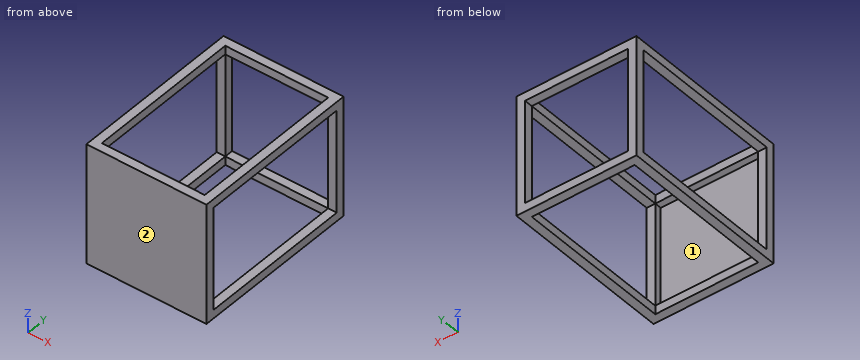
Autodesk Inventor part; units mm, degrees
ref_plane "YZ Plane" through (0, 0, 0) normal (1, 0, 0) x (0, 1, 0)
ref_plane "XZ Plane" through (0, 0, 0) normal (0, 1, 0) x (-1, 0, 0)
ref_plane "XY Plane" through (0, 0, 0) normal (0, 0, 1) x (1, 0, 0)
sketch "Sketch1" plane through (0, 0, 0) normal (0, 0, 1) x (1, 0, 0)
  point P0 (0, 0)
sketch "Sketch2" plane through (0, 0, 0) normal (0, 1, 0) x (-1, 0, 0)
  line L0 (-300, 300) -> (300, 300)
  line L1 (300, 300) -> (300, -300)
  line L2 (300, -300) -> (-300, -300)
  line L3 (-300, -300) -> (-300, 300)
  line L4 (-300, 300) -> (300, -300) construction
  line L5 (300, 300) -> (-300, -300) construction
  line L6 (350, 350) -> (-350, 350)
  line L7 (-350, 350) -> (-350, -350)
  line L8 (-350, -350) -> (350, -350)
  line L9 (350, -350) -> (350, 350)
  line L10 (350, 350) -> (-350, -350) construction
  line L11 (-350, 350) -> (350, -350) construction
  line L12 (-300, 300) -> (-350, 300)
  line L13 (-350, 300) -> (-350, 350)
  line L14 (-350, 350) -> (-300, 350)
  line L15 (-300, 350) -> (-300, 300)
  line L16 (300, 300) -> (350, 300)
  line L17 (350, 300) -> (350, 350)
  line L18 (350, 350) -> (300, 350)
  line L19 (300, 350) -> (300, 300)
  line L20 (350, -350) -> (300, -350)
  line L21 (300, -350) -> (300, -300)
  line L22 (300, -300) -> (350, -300)
  line L23 (350, -300) -> (350, -350)
  line L24 (-350, -350) -> (-300, -350)
  line L25 (-300, -350) -> (-300, -300)
  line L26 (-300, -300) -> (-350, -300)
  line L27 (-350, -300) -> (-350, -350)
  point P0 (0, 0)
  dimension "d0" = 600
  dimension "d1" = 600
  dimension "d2" = 700
  dimension "d3" = 700
extrude "Extrusion1" add sketch "Sketch2" along normal blind 10 contours L0 L1 L2 L3
extrude "Extrusion2" add sketch "Sketch2" along normal blind 50 contours L15 L6 L19 L0 | L3 L26 L7 L12 | L12 L7 L6 L15 | L16 L9 L22 L1 | L19 L6 L9 L16 | L2 L21 L8 L25 | L25 L8 L7 L26 | L22 L9 L8 L21
extrude "Extrusion3" add sketch "Sketch2" along normal blind 1000 contours L12 L7 L6 L15 | L19 L6 L9 L16 | L25 L8 L7 L26 | L22 L9 L8 L21
sketch3d "3D Sketch1"
sketch "Sketch3" plane through (-300, 50, 300) normal (1, 0, 0) x (0, 0, -1)
  line L0 (-50, -50) -> (-50, 950)
  line L1 (0, 0) -> (0, 950)
  line L2 (-50, 950) -> (0, 950)
  line L3 (0, 950) -> (0, 900)
  line L4 (0, 900) -> (-50, 900)
  line L5 (-50, 900) -> (-50, 950)
  point P0 (300, -50)
  dimension "d13" = 50
sketch "Sketch4" plane through (-300, 50, 300) normal (1, 0, 0) x (0, 0, -1)
  point P0 (300, -50)
extrude "Extrusion4" add sketch "Sketch3" along normal up to surface (600 mm away)
sketch "Sketch5" plane through (300, 50, -300) normal (0, 0, 1) x (1, 0, 0)
  line L0 (50, 950) -> (-650, 950)
  line L1 (0, 0) -> (0, 900)
  line L2 (50, 950) -> (0, 950)
  line L3 (0, 950) -> (0, 900)
  line L4 (0, 900) -> (50, 900)
  line L5 (50, 900) -> (50, 950)
  point P0 (-300, -50)
extrude "Extrusion5" add sketch "Sketch5" along normal up to surface (600 mm away)
sketch "Sketch6" plane through (-300, 50, -350) normal (1, 0, 0) x (0, 0, -1)
  line L0 (-50, 0) -> (-50, 950)
  line L1 (0, 0) -> (0, 950)
  line L2 (-50, 950) -> (0, 950)
  line L3 (0, 950) -> (0, 900)
  line L4 (0, 900) -> (-50, 900)
  line L5 (-50, 900) -> (-50, 950)
  point P0 (-350, -50)
  dimension "d18" = 50
extrude "Extrusion6" add sketch "Sketch6" along normal up to surface (600 mm away)
sketch "Sketch7" plane through (-350, 1000, -300) normal (0, 0, 1) x (1, 0, 0)
  line L0 (0, -950) -> (0, 0)
  line L1 (50, -950) -> (50, -50)
  line L2 (0, 0) -> (50, 0)
  line L3 (50, 0) -> (50, -50)
  line L4 (50, -50) -> (0, -50)
  line L5 (0, -50) -> (0, 0)
  point P0 (350, -1000)
extrude "Extrusion7" add sketch "Sketch7" along normal up to surface (600 mm away)
properties part number "Frame"
Could you check a few things on this model? Use its own coordinates, in mm. Face numbers are marked on the shaded views. Round coordinates to 2 decimals unless told otherwise and drop trailing zeros. Order: outer loops, then holes, each group sorted by start corner. A loop starts at its lowest first (then second) coordinate and runs counter-clockwise, first axis right, second up. Notation, with made-up numbers: M 27,-23.75 L 74,-23.75 A8 cw 74,-12.75 Z; hole C 11.5,59.25 d11. An arc over 180 degrees is marked long. One line per question, with ' | ' between items. Start each with the question number.
(1) Please list where these lines run through material, in increasing order: line 1 along X through (y, z) = (318, 321.5); line 2 along Y through (x, z) = (319, -275).
(2) Suppose I cut it at B-B on x = 179. List the corners of the cut face in (y, z) for me.
(3) Thinking about a two-plate mould opening in Z: for the marked faces 1 and 2, which applies, +Z half, -Z half, draft (parallel to the pull), parting line (faces both ways), or undercut?
(4) For P1, Ø25, axis at x = 316, z = 59, coming from the -Y side; P2, Ø12, axis at x = 179, z = 87, coming from the +Y side, each with a flat end and sliding along its axis, tell me the tip position at first contact or that it passes through.
(5) Suppose I cut it at A-A on y = 777. List the corners of the cut face in (x, z) for me.
(6) Suppose I cut it at C-C on z = 45. List the corners of the cut face in (x, y) for me, then the cut area to 3 significant figures.
Geometry results:
1) line 1: -350 to -300, 300 to 350 | line 2: 0 to 50, 950 to 1000
2) outline: M 0,-350 L 50,-350 L 50,-300 L 10,-300 L 10,300 L 50,300 L 50,350 L 0,350 Z; M 950,-350 L 1000,-350 L 1000,-300 L 950,-300 Z; M 950,300 L 1000,300 L 1000,350 L 950,350 Z
3) face 1: undercut | face 2: draft
4) P1: y = 0 | P2: y = 10
5) outline: M -350,-350 L -300,-350 L -300,-300 L -350,-300 Z; M -350,300 L -300,300 L -300,350 L -350,350 Z; M 300,-350 L 350,-350 L 350,-300 L 300,-300 Z; M 300,300 L 350,300 L 350,350 L 300,350 Z
6) outline: M -350,0 L 350,0 L 350,50 L 300,50 L 300,10 L -300,10 L -300,50 L -350,50 Z; M -350,950 L -300,950 L -300,1000 L -350,1000 Z; M 300,950 L 350,950 L 350,1000 L 300,1000 Z | area: 16,000 mm²
